from build123d import *

# Parameters (mm, degrees)
SKETCH1_W           = 55.88
SKETCH1_H           = 12.7
BOSS_EXTRUDE1_DEPTH = 5.08
SKETCH2_W           = 30.48
SKETCH2_H           = 6.35
CUT_EXTRUDE1_DEPTH  = 5.08
FILLET1_R           = 5.08
SKETCH3_W           = 2.54
SKETCH3_H           = 5.08
BOSS_EXTRUDE2_DEPTH = 10.16


with BuildPart() as part:
    # Sketch1 → Boss-Extrude1 (new body)
    with BuildSketch(Plane(origin=(0, 0, 0), x_dir=(1, 0, 0), z_dir=(0, 1, 0))):
        Rectangle(SKETCH1_W, SKETCH1_H)
    extrude(amount=BOSS_EXTRUDE1_DEPTH)

    # Sketch2 → Cut-Extrude1 (cut)
    with BuildSketch(Plane(origin=(0, 5.08, 0), x_dir=(1, 0, 0), z_dir=(0, 1, 0))):
        with Locations((0, 3.175)):
            Rectangle(SKETCH2_W, SKETCH2_H)
    extrude(amount=-CUT_EXTRUDE1_DEPTH, mode=Mode.SUBTRACT)

    # Fillet1
    fillet1_edges = [part.edges().sort_by_distance(p)[0] for p in [
        (27.94, 2.54, 6.35),
        (-27.94, 2.54, 6.35),
        (-27.94, 2.54, -6.35),
        (27.94, 2.54, -6.35),
    ]]
    fillet(fillet1_edges, radius=FILLET1_R)

    # Sketch3 → Boss-Extrude2 (add)
    with BuildSketch(Plane(origin=(0, 0, -6.35), x_dir=(-1, 0, 0), z_dir=(0, 0, -1))):
        with Locations((17.382512253, 2.54)):
            Rectangle(SKETCH3_W, SKETCH3_H)
    boss_extrude2 = extrude(amount=BOSS_EXTRUDE2_DEPTH)

    # Mirror1: Boss-Extrude2 across plane
    add(boss_extrude2.mirror(Plane(origin=(0, 0, 0), x_dir=(0, 0, 1), z_dir=(1, 0, 0))))


solid = part.part
Geometry: final body of the model. Coordinates: model frame, mm. A direction names the side the tool comes from. Round coordinates to 2 decimals unless told otherwise and drop trailing zeros. Loops run counter-clockwise (first coordinate to the right, second up) from the corner with the lowest first, then second, coordinate; pieces in that order, holes last. Notation, with made-up numbers: M -7,59.5 L 44,59.5 A15 ccw 44,77.5 Z; hole C -1.75,58 d2. An arc over 180 degrees is marked long. One line per question, with ' | ' between items.
(1) Cut plane B-B on y = 1.75. Return the cut outline in (x, z).
Check result:
outline: M -27.94,-1.27 A5.08 ccw -22.86,-6.35 L -18.65,-6.35 L -18.65,-16.51 L -16.11,-16.51 L -16.11,-6.35 L -15.24,-6.35 L -15.24,0 L 15.24,0 L 15.24,-6.35 L 16.11,-6.35 L 16.11,-16.51 L 18.65,-16.51 L 18.65,-6.35 L 22.86,-6.35 A5.08 ccw 27.94,-1.27 L 27.94,1.27 A5.08 ccw 22.86,6.35 L -22.86,6.35 A5.08 ccw -27.94,1.27 Z
(2) Cut plane C-C on x = 14.5. Return the cut outline in (y, z), plus the area to 3 significant figures.
Check result:
outline: M 0,0 L 5.08,0 L 5.08,6.35 L 0,6.35 Z | area: 32.3 mm2
(3) Pull-direction query (X, two-part tool) for faces 4 (the flat face through (-16.113, 3, -11)), 5 (the cylindrical face through (26.412, 2.576, 4.901)), 6 (the flat face through (0, 3, 0)), 7 (the flat face through (-21, 3, -6.35)); classes: +X half, -X half, draft (parallel to the pull), parting line (faces both ways), or undercut.
Check result:
face 4: undercut | face 5: +X half | face 6: undercut | face 7: draft
(4) Cut plane A-A on z = -8.5. Return the cut outline in (x, y).
Check result:
outline: M -18.65,0 L -16.11,0 L -16.11,5.08 L -18.65,5.08 Z; M 16.11,0 L 18.65,0 L 18.65,5.08 L 16.11,5.08 Z
(5) Cut plane D-D on z = -4. Return the cut outline in (x, y), plus the area to 3 significant figures.
Check result:
outline: M -27.14,0 L -15.24,0 L -15.24,5.08 L -27.14,5.08 Z; M 15.24,0 L 27.14,0 L 27.14,5.08 L 15.24,5.08 Z | area: 121 mm2
(6) Access query for faces 1 (the flat face through (21, 3, -6.35)), 2 (the flat face through (-18.653, 3, -11)), 3 (the flat face through (16.113, 3, -11)). Directions: +Z, -Z, +X, -X, +Y, -Y. A direction counts if a zero-diameter tool reaches every point of the face in a straight line with its end or side. Return the directions, or none.
Check result:
face 1: -Z, +X, +Y, -Y | face 2: -Z, -X, +Y, -Y | face 3: -Z, +Y, -Y
(7) Contact query for flat-ended pins moving along their axis: P1, Ø1.5, axis at y = 1.5, z = -10, coming from the +X side; P2, Ø1, axis at x = 15.5, y = 4, coming from the -Z side; P3, Ø3, axis at x = 19.5, z = -14, coming from the -Y side; P4, Ø1.5, axis at y = 2.5, z = -12, coming from the -X side. Output: stop coordinate, or through.
Check result:
P1: stops at x = 18.65 | P2: stops at z = -6.35 | P3: stops at y = 0 | P4: stops at x = -18.65
(8) Material intervals for line 1 along X through (y, z) = (2.5, -6.5); line 2 along Z through (x, y) = (-10, 3.4); line 3 along Z through (x, y) = (21.5, 4.4), sorted ascending. Write a range as from..to.
Check result:
line 1: x = -18.65..-16.11, 16.11..18.65 | line 2: z = 0..6.35 | line 3: z = -6.35..6.35
